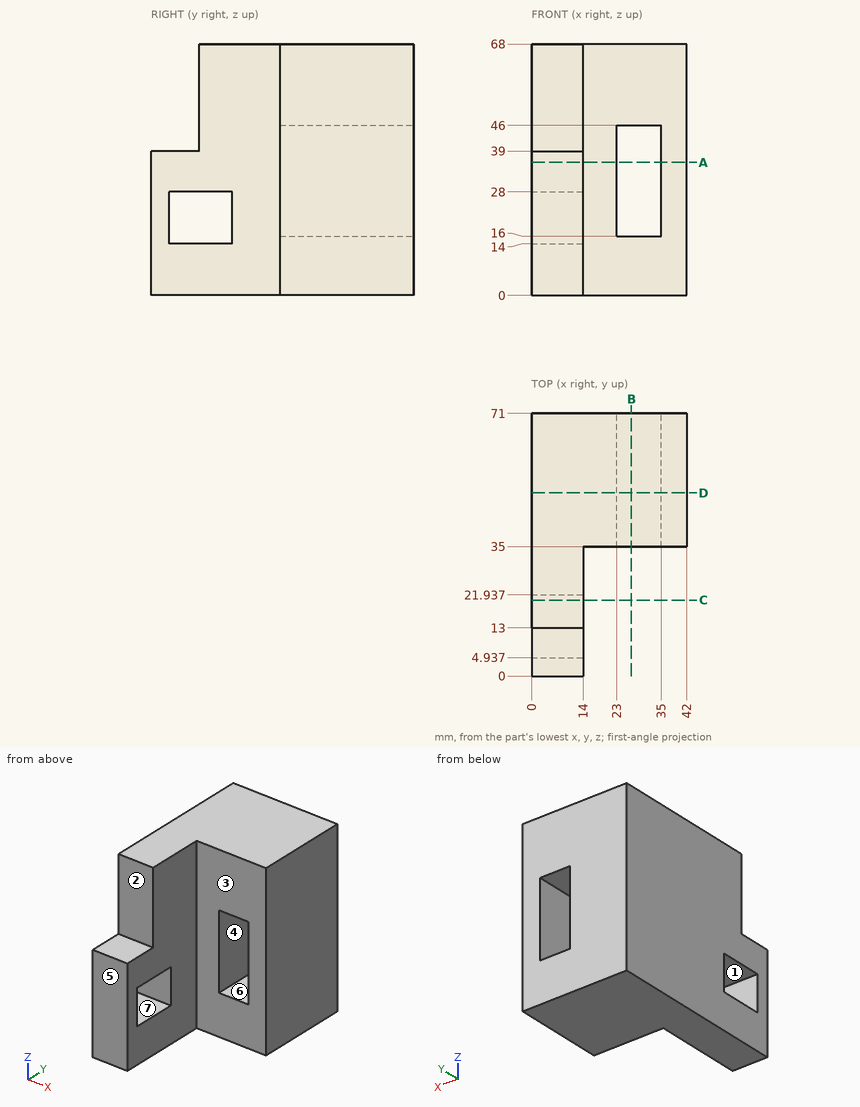
Answer from the drawing. Dimensions are ordinates in mm from the lowest x, y and z of the part. A direction names the side the tool comes from. Give positions to 0.01 mm unless a question says otherwise; leave off trailing zeros. Loops run counter-clockwise (first coordinate to the right, second up) from the corner with the lowest first, then second, coordinate; pieces in that order, holes last. Notation, with made-up numbers: (47, 42.25) -> (104, 42.25) arc R19 cw to (104, 55.25) -> close; hole circle Ø11 at (-3, -1.75). An arc over 180 degrees is marked (long way). Use a Markdown table: item, result.
Q1. Each of these flat-tipped pins is pushed along its axis until it touches: pin 1 (4 mm diameter, centred on x = 9, z = 50, fed in from -Y); pin 2 (4 mm diameter, centred on y = 9.5, z = 26.5, fed in from +X); pin 3 (14.5 mm diameter, centred on x = 4.5, y = 4.5, fed in from +Z). Where does it stop, or does it pass through?
Solved:
| item | result |
|---|---|
| pin 1 | stops at y = 13 |
| pin 2 | stops at x = 14 |
| pin 3 | stops at z = 39 |
Q2. Section A-A, the plane z = 36 is taken. Determine the outline of the cut face in (x, y), then the cut area to 3 significant figures.
Solved:
| item | result |
|---|---|
| outline | (0, 0) -> (14, 0) -> (14, 35) -> (23, 35) -> (23, 71) -> (0, 71) -> close; (35, 35) -> (42, 35) -> (42, 71) -> (35, 71) -> close |
| area | 1,570 mm^2 |
Q3. Section D-D, the plane y = 49.5 is taken. Determine the outline of the cut face in (x, z).
Solved:
| item | result |
|---|---|
| outline | (0, 0) -> (42, 0) -> (42, 68) -> (0, 68) -> close; hole (23, 16) -> (35, 16) -> (35, 46) -> (23, 46) -> close |
Q4. Find the intervals of material crossed by line 1 along Z through (x, y) = (9.5, 15); line 2 along Z through (x, y) = (31.5, 49); line 3 along Y through (x, z) = (12, 17.5), in increasing order.
Solved:
| item | result |
|---|---|
| line 1 | z = 0 to 14, 28 to 68 |
| line 2 | z = 0 to 16, 46 to 68 |
| line 3 | y = 0 to 4.94, 21.94 to 71 |
Q5. Section C-C, the plane y = 20.5 is taken. Determine the outline of the cut face in (x, z).
Solved:
| item | result |
|---|---|
| outline | (0, 0) -> (14, 0) -> (14, 14) -> (0, 14) -> close; (0, 28) -> (14, 28) -> (14, 68) -> (0, 68) -> close |
Q6. A tool of negligible diameter and unlimited length cuts with its end or side. For the marked faces 1, 2, 3 and 4, from which of +Z, -Z, +X, -X, +Y, -Y can it reach the whole face along a straight path? Write none if from no direction.
Solved:
| item | result |
|---|---|
| face 1 | +X, -X |
| face 2 | +Z, +X, -X, -Y |
| face 3 | +Z, -Z, +X, -Y |
| face 4 | +Y, -Y |
Q7. Determine the mould class of the marked faces 5, 6 and 7 for opening direction Y: pulls with the +Y half, pulls with the -Y half, needs draft (parallel to the pull), parting line crosses it, or undercut.
Solved:
| item | result |
|---|---|
| face 5 | pulls with the -Y half |
| face 6 | needs draft |
| face 7 | undercut |
Q8. Section B-B, the plane x = 27 is taken. Determine the outline of the cut face in (y, z), then the cut area to 3 significant figures.
Solved:
| item | result |
|---|---|
| outline | (35, 0) -> (71, 0) -> (71, 16) -> (35, 16) -> close; (35, 46) -> (71, 46) -> (71, 68) -> (35, 68) -> close |
| area | 1,370 mm^2 |
